```python
from build123d import *

# Parameters (mm, degrees)
F0_W     = 14.4847853028
F0_H     = 313
F1_DEPTH = 10
F2_R     = 4.99999


# Not quite as in the source:
# - a fillet or chamfer is up to 0.001 mm smaller than in the source, because OpenCascade refuses the exact size


with BuildPart() as f1:
    # F0 (on Right) → F1 (new body)
    with BuildSketch(Plane.YZ):
        with Locations((-49.3265521361, 156.5)):
            Rectangle(F0_W, F0_H)
        Polygon((-42.0841594847, 313), (-42.0841594847, 0), (-23.5623567487, 0), (-23.5623567487, 356.9950582001), (-56.5689447875, 313), align=None)
    extrude(amount=F1_DEPTH)

    # F2 (radius 5 in the source; OpenCascade refuses exactly that, so slightly less here)
    f2_edges = [f1.edges().sort_by_distance(p)[0] for p in [
        (10, -40.065651, 334.997529),
        (0, -40.065651, 334.997529),
    ]]
    fillet(f2_edges, radius=F2_R)


solid = f1.part
```
Could you check a few things on this model? Use its own coordinates, in mm. Coordinates: 2 decimals unless noted, no trailing zeros. Order: outer loops, then holes, each group sorted by start corner. A loop starts at its lowest first (then second) coordinate and runs counter-clockwise, first axis right, second up. Notation, with made-up numbers: M -39.5,10.25 L -12.5,10.25 A25 cw -12.5,27.25 Z; hole C 89.25,67.25 d11. An arc over 180 degrees is marked long. Use a Markdown table: item, result. Add a question column.
Q1. I want a section at A-A on x = 7.5. List the corners of the cut face in (y, z) for me.
Q2. If I drill on L1, parallel to Z at x = 4.25, y = -48.5; L2, parallel to Z at x = 1, y = -25; L3, parallel to Y at x = 4.25, z = 339.5, over which ranges is the centre line in solid material (lowest first)?
Q3. I'm going to push a flat-ended pin straight in: pin 1 (4 mm diameter, centred on x = 2.5, y = -28.5, fed in from +Z). Where does the tip first touch, or does it pass through?
Checked values:
| question | item | result |
|---|---|---|
| 1 | outline | M -56.57,0 L -23.56,0 L -23.56,355.88 L -56.57,311.88 Z |
| 2 | L1 | 0 to 323.66 |
| 2 | L2 | 0 to 351.75 |
| 2 | L3 | -36.62 to -23.56 |
| 3 | pin 1 | z = 352.36 |
